Check sheet for the modelled part. Datum: model origin and axes. Units: mm. A direction names the side the tool comes from. Give positions to 0.01 mm unless a question says otherwise; leave off trailing zeros. Write each loop counter-clockwise with the first axis right and the second up, starting at its lowest first coordinate (ties: lowest second). Pieces come first, ordered by that corner, then holes. Notation, with made-up numbers: M 52.5,-27.75 L 75.5,-27.75 A12 ccw 75.5,-18.75 Z; hole C 55.5,47.5 d10. An arc over 180 degrees is marked long. One line per item, written item: value. Start each with the question number.
Autodesk Inventor part; units mm, degrees
ref_plane "YZ Plane" through (0, 0, 0) normal (1, 0, 0) x (0, 1, 0)
ref_plane "XZ Plane" through (0, 0, 0) normal (0, 1, 0) x (-1, 0, 0)
ref_plane "XY Plane" through (0, 0, 0) normal (0, 0, 1) x (1, 0, 0)
sketch "스케치1" plane through (0, 0, 0) normal (0, 0, 1) x (1, 0, 0)
  circle A0 centre (0, 0) radius 19.4
  circle A1 centre (10.6066, 10.6066) radius 1.65
  circle A2 centre (0, 0) radius 11
  circle A3 centre (-10.6066, 10.6066) radius 1.65
  circle A4 centre (-10.6066, -10.6066) radius 1.65
  circle A5 centre (10.6066, -10.6066) radius 1.65
  dimension "d1" = 22
  dimension "d5" = 360
extrude "돌출1" add sketch "스케치1" along normal blind 4.8
sketch "스케치2" plane through (0, 0, 4.8) normal (0, 0, 1) x (1, 0, 0)
  circle A0 centre (0, 0) radius 19.4
  circle A1 centre (10.6066, -10.6066) radius 1.65
  circle A2 centre (-10.6066, -10.6066) radius 1.65
  circle A3 centre (-10.6066, 10.6066) radius 1.65
  circle A4 centre (0, 0) radius 11
  circle A5 centre (10.6066, 10.6066) radius 1.65
  line L0 (10.6066, 10.6066) -> (8.8388, 8.8388)
  line L1 (10.6066, 10.6066) -> (13.1066, 10.6066) construction
  line L2 (7.8182, 9.8595) -> (8.5654, 12.6478)
  line L3 (8.5654, 12.6478) -> (11.3537, 13.395)
  line L4 (11.3537, 13.395) -> (13.395, 11.3537)
  line L5 (13.395, 11.3537) -> (12.6478, 8.5654)
  line L6 (12.6478, 8.5654) -> (9.8595, 7.8182)
  line L7 (9.8595, 7.8182) -> (7.8182, 9.8595)
  line L8 (-10.6066, 10.6066) -> (-10.6066, 13.1066) construction
  line L9 (-13.395, 11.3537) -> (-11.3537, 13.395)
  line L10 (-11.3537, 13.395) -> (-8.5654, 12.6478)
  line L11 (-8.5654, 12.6478) -> (-7.8182, 9.8595)
  line L12 (-7.8182, 9.8595) -> (-9.8595, 7.8182)
  line L13 (-12.6478, 8.5654) -> (-13.395, 11.3537)
  line L14 (-9.8595, 7.8182) -> (-12.6478, 8.5654)
  line L15 (-10.6066, -10.6066) -> (-13.1066, -10.6066) construction
  line L16 (-11.3537, -13.395) -> (-13.395, -11.3537)
  line L17 (-13.395, -11.3537) -> (-12.6478, -8.5654)
  line L18 (-12.6478, -8.5654) -> (-9.8595, -7.8182)
  line L19 (-9.8595, -7.8182) -> (-7.8182, -9.8595)
  line L20 (-8.5654, -12.6478) -> (-11.3537, -13.395)
  line L21 (-7.8182, -9.8595) -> (-8.5654, -12.6478)
  line L22 (10.6066, -10.6066) -> (10.6066, -13.1066) construction
  line L23 (13.395, -11.3537) -> (11.3537, -13.395)
  line L24 (11.3537, -13.395) -> (8.5654, -12.6478)
  line L25 (8.5654, -12.6478) -> (7.8182, -9.8595)
  line L26 (7.8182, -9.8595) -> (9.8595, -7.8182)
  line L27 (12.6478, -8.5654) -> (13.395, -11.3537)
  line L28 (9.8595, -7.8182) -> (12.6478, -8.5654)
  point P0 (-8.8388, 8.8388)
  point P1 (-8.8388, -8.8388)
  point P2 (8.8388, -8.8388)
  dimension "d9" = 2.5
  dimension "d10" = 135
  dimension "d13" = 360
extrude "돌출2" cut sketch "스케치2" against normal blind 3 contours A1 | A2 | A3 | A5 | L7 L2 L3 L4 L5 L6 | L9 L10 L11 L12 L14 L13 | L16 L17 L18 L19 L21 L20 | L23 L24 L25 L26 L28 L27
sketch "스케치3" plane through (0, 0, 4.8) normal (0, 0, 1) x (1, 0, 0)
  circle A0 centre (0, 0) radius 16
  circle A1 centre (0, 0) radius 22.4
  line L0 (-7.8182, 9.8595) -> (-9.8595, 7.8182)
  line L1 (-9.8595, 7.8182) -> (-12.6478, 8.5654)
  line L2 (-12.6478, 8.5654) -> (-13.395, 11.3537)
  line L3 (-13.395, 11.3537) -> (-11.3537, 13.395)
  line L4 (-11.3537, 13.395) -> (-8.5654, 12.6478)
  line L5 (-8.5654, 12.6478) -> (-7.8182, 9.8595)
  line L6 (-9.8595, -7.8182) -> (-7.8182, -9.8595)
  line L7 (-7.8182, -9.8595) -> (-8.5654, -12.6478)
  line L8 (-8.5654, -12.6478) -> (-11.3537, -13.395)
  line L9 (-11.3537, -13.395) -> (-13.395, -11.3537)
  line L10 (-13.395, -11.3537) -> (-12.6478, -8.5654)
  line L11 (-12.6478, -8.5654) -> (-9.8595, -7.8182)
  line L12 (13.395, 11.3537) -> (12.6478, 8.5654)
  line L13 (12.6478, 8.5654) -> (9.8595, 7.8182)
  line L14 (9.8595, 7.8182) -> (7.8182, 9.8595)
  line L15 (7.8182, 9.8595) -> (8.5654, 12.6478)
  line L16 (8.5654, 12.6478) -> (11.3537, 13.395)
  line L17 (11.3537, 13.395) -> (13.395, 11.3537)
  line L18 (7.8182, -9.8595) -> (9.8595, -7.8182)
  line L19 (9.8595, -7.8182) -> (12.6478, -8.5654)
  line L20 (12.6478, -8.5654) -> (13.395, -11.3537)
  line L21 (13.395, -11.3537) -> (11.3537, -13.395)
  line L22 (11.3537, -13.395) -> (8.5654, -12.6478)
  line L23 (8.5654, -12.6478) -> (7.8182, -9.8595)
  circle A2 centre (0, 0) radius 19.4
  circle A3 centre (0, 0) radius 11
  point P0 (-9.4762, 12.8919)
  point P1 (9.4762, 12.8919)
  point P2 (12.8919, 9.4762)
  point P3 (12.8919, -9.4762)
  point P4 (9.4762, -12.8919)
  point P5 (-9.4762, -12.8919)
  point P6 (-12.8919, -9.4762)
  point P7 (-12.8919, 9.4762)
  dimension "d17" = 32
  dimension "d18" = 6.4
extrude "돌출3" add sketch "스케치3" along normal blind 7 contours A1 | A2
chamfer "모따기1" distance 3 angle 45 1 edges at (-19.4, 0, 4.8)
sketch "스케치4" plane through (0, 0, 4.8) normal (0, 0, 1) x (1, 0, 0)
  circle A0 centre (0, 0) radius 11
  arc A1 (12.8919, -9.4762) -> (12.8919, 9.4762) centre (0, 0) ccw
  line L0 (12.8919, 9.4762) -> (12.6478, 8.5654)
  line L1 (12.6478, 8.5654) -> (9.8595, 7.8182)
  line L2 (9.8595, 7.8182) -> (7.8182, 9.8595)
  line L3 (7.8182, 9.8595) -> (8.5654, 12.6478)
  line L4 (8.5654, 12.6478) -> (9.4762, 12.8919)
  arc A2 (9.4762, 12.8919) -> (-9.4762, 12.8919) centre (0, 0) ccw
  line L5 (-9.4762, 12.8919) -> (-8.5654, 12.6478)
  line L6 (-8.5654, 12.6478) -> (-7.8182, 9.8595)
  line L7 (-7.8182, 9.8595) -> (-9.8595, 7.8182)
  line L8 (-9.8595, 7.8182) -> (-12.6478, 8.5654)
  line L9 (-12.6478, 8.5654) -> (-12.8919, 9.4762)
  arc A3 (-12.8919, 9.4762) -> (-12.8919, -9.4762) centre (0, 0) ccw
  line L10 (-12.8919, -9.4762) -> (-12.6478, -8.5654)
  line L11 (-12.6478, -8.5654) -> (-9.8595, -7.8182)
  line L12 (-9.8595, -7.8182) -> (-7.8182, -9.8595)
  line L13 (-7.8182, -9.8595) -> (-8.5654, -12.6478)
  line L14 (-8.5654, -12.6478) -> (-9.4762, -12.8919)
  arc A4 (-9.4762, -12.8919) -> (9.4762, -12.8919) centre (0, 0) ccw
  line L15 (9.4762, -12.8919) -> (8.5654, -12.6478)
  line L16 (8.5654, -12.6478) -> (7.8182, -9.8595)
  line L17 (7.8182, -9.8595) -> (9.8595, -7.8182)
  line L18 (9.8595, -7.8182) -> (12.6478, -8.5654)
  line L19 (12.6478, -8.5654) -> (12.8919, -9.4762)
  circle A5 centre (0, 0) radius 11.4
  line L20 (9.8595, 7.8182) -> (9.0168, 6.9755)
  line L21 (8.8388, 8.8388) -> (8.4116, 8.4116)
  line L22 (7.8182, 9.8595) -> (6.9755, 9.0168)
  line L23 (-7.8182, 9.8595) -> (-6.9755, 9.0168)
  line L24 (-9.8595, 7.8182) -> (-9.0168, 6.9755)
  line L25 (-9.8595, -7.8182) -> (-9.0168, -6.9755)
  line L26 (-7.8182, -9.8595) -> (-6.9755, -9.0168)
  line L27 (7.8182, -9.8595) -> (6.9755, -9.0168)
  line L28 (9.8595, -7.8182) -> (9.0168, -6.9755)
  dimension "d24" = 0.4
  dimension "d27" = 360
extrude "돌출4" cut sketch "스케치4" against normal blind 7 contours A5
extrude "돌출5" cut sketch "스케치4" against normal up to surface (3 mm away) contours L17 L27 A5 L28 | L20 A5 L22 L2 | L26 L12 L25 A5 | A5 L24 L7 L23
sketch "스케치5" plane through (0, 0, 11.8) normal (0, 0, 1) x (1, 0, 0)
  circle A0 centre (0, 0) radius 22.4
  circle A1 centre (0, 0) radius 20.4
  dimension "d33" = 2
extrude "돌출6" cut sketch "스케치5" against normal blind 10
sketch "스케치6" plane through (0, 0, 4.8) normal (0, 0, 1) x (1, 0, 0)
  circle A0 centre (0, 0) radius 12.2
  dimension "d36" = 24.4
extrude "돌출7" cut sketch "스케치6" against normal blind 0.8
chamfer "모따기2" distance 0.8 angle 45 4 edges at (12.2, 0, 4) (0, -12.2, 4) (0, 12.2, 4) (-12.2, 0, 4)
sketch "스케치7" plane through (0, 0, 11.8) normal (0, 0, 1) x (1, 0, 0)
  circle A0 centre (0, 0) radius 20.4
  line L0 (-13.395, 11.3537) -> (-11.3537, 13.395)
  line L1 (-11.3537, 13.395) -> (-9.4762, 12.8919)
  arc A1 (9.4762, 12.8919) -> (-9.4762, 12.8919) centre (0, 0) ccw
  line L2 (9.4762, 12.8919) -> (11.3537, 13.395)
  line L3 (11.3537, 13.395) -> (13.395, 11.3537)
  line L4 (13.395, 11.3537) -> (12.8919, 9.4762)
  arc A2 (12.8919, -9.4762) -> (12.8919, 9.4762) centre (0, 0) ccw
  line L5 (12.8919, -9.4762) -> (13.395, -11.3537)
  line L6 (13.395, -11.3537) -> (11.3537, -13.395)
  line L7 (11.3537, -13.395) -> (9.4762, -12.8919)
  arc A3 (-9.4762, -12.8919) -> (9.4762, -12.8919) centre (0, 0) ccw
  line L8 (-9.4762, -12.8919) -> (-11.3537, -13.395)
  line L9 (-11.3537, -13.395) -> (-13.395, -11.3537)
  line L10 (-13.395, -11.3537) -> (-12.8919, -9.4762)
  arc A4 (-12.8919, 9.4762) -> (-12.8919, -9.4762) centre (0, 0) ccw
  line L11 (-12.8919, 9.4762) -> (-13.395, 11.3537)
  circle A5 centre (10.6066, 10.6066) radius 1.65
  line L12 (10.6066, 10.6066) -> (13.118, 9.9337)
  line L13 (12.7295, 8.4837) -> (9.8296, 7.7067)
  line L14 (7.7067, 9.8296) -> (8.4837, 12.7295)
  line L15 (8.4837, 12.7295) -> (11.3836, 13.5065)
  line L16 (11.3836, 13.5065) -> (13.5065, 11.3836)
  line L17 (13.5065, 11.3836) -> (12.7295, 8.4837)
  line L18 (7.7067, 9.8296) -> (6.6452, 8.7681)
  line L19 (6.6452, 8.7681) -> (8.7681, 6.6452)
  line L20 (8.7681, 6.6452) -> (9.8296, 7.7067)
  point P0 (9.3724, 12.9676)
  point P1 (12.9676, 9.3724)
  dimension "d42" = 2.6
extrude "돌출8" cut sketch "스케치7" against normal up to surface (10 mm away) contours L15 L16 L17 L12 L4 L3 L2 A1 | A1 L2 L3 L4 A2 L17 L13 L20 L19 L18 L14 L15 | L17 A2 L4 L12
pattern_circular "원형 패턴1" count 4 over 360 about axis through (0, 0, 4.8) along (0, 0, -1) of "돌출8"
fillet "모깎기1" radius 2 8 edges at (12.9676, 9.3724, 8.3) (9.3724, 12.9676, 8.3) (12.9676, -9.3724, 8.3) (9.3724, -12.9676, 8.3) (-9.3724, -12.9676, 8.3) (-12.9676, -9.3724, 8.3) (-12.9676, 9.3724, 8.3) (-9.3724, 12.9676, 8.3)
properties part number "ShaftLock_B"
1) Tool access check on faces 1 (the cylindrical face through (11.49, -12, 0.89)), 2 (the flat face through (-11.3, -8.1, 3.3)). Record the directions out of +Z, -Z, +X, -X, +Y, -Y that give a thin tool (end or side, any length) a straight path to the whole face; none if there is none.
2) Cross-section at C-C (z = 0.75). Record the boundary of the cut face in (x, y).
3) Material ranges on L1, parallel to Y at x = 10, z = 1.5; L2, parallel to Y at x = -6.5, z = 4.25; L3, parallel to X at y = 7, z = 7.5, recorded low to high. Write a range as from..to.
4) Draft check along X on faces 3 (the cylindrical face through (9.41, -18.1, 7.36)), 4 (the flat face through (15, -6, 11.8)), 5 (the flat face through (0, -13, 4.8)). Enter one of: released by +X, released by -X, zero draft, split by the parting line, or undercut.
5) Gauge pin test, flat ends, axial feed: pin 1 (3 mm diameter, centred on x = 13, y = 3.5, fed in from +Z); pin 2 (4 mm diameter, centred on y = 15, z = 10, fed in from -X); pin 3 (2 mm diameter, centred on x = 8, z = 4, fed in from -Y). Record the tip position at first contact, or that the pin passes through.
6) Cross-section at B-B (z = 11). Record the boundary of the cut face in (x, y).
Data:
1. face 1: +Z, -Z
1. face 2: +Z
2. outline: C 0,0 d38.8; hole C -10.61,-10.61 d3.3; hole C -10.61,10.61 d3.3; hole C 0,0 d22.8; hole C 10.61,-10.61 d3.3; hole C 10.61,10.61 d3.3
3. L1: y = -16.62..-12.14, -9.07..-5.47, 5.47..9.07, 12.14..16.62
3. L2: y = -19.34..-9.67, 9.67..19.34
3. L3: x = -19.16..-14.39, 14.39..19.16
4. face 3: split by the parting line
4. face 4: zero draft
4. face 5: undercut
5. pin 1: stops at z = 4.8
5. pin 2: stops at x = -15.72
5. pin 3: stops at y = -19.16
6. outline: C 0,0 d40.8; hole M -13.51,-11.38 L -11.38,-13.51 L -10.26,-13.2 A2 cw -8.66,-13.45 A16 ccw 8.66,-13.45 A2 cw 10.26,-13.2 L 11.38,-13.51 L 13.51,-11.38 L 13.2,-10.26 A2 cw 13.45,-8.66 A16 ccw 13.45,8.66 A2 cw 13.2,10.26 L 13.51,11.38 L 11.38,13.51 L 10.26,13.2 A2 cw 8.66,13.45 A16 ccw -8.66,13.45 A2 cw -10.26,13.2 L -11.38,13.51 L -13.51,11.38 L -13.2,10.26 A2 cw -13.45,8.66 A16 ccw -13.45,-8.66 A2 cw -13.2,-10.26 Z
